The model under review builds one solid part; all positions refer to its coordinate system, in mm. A direction names the side the tool comes from. Give positions to 0.01 mm unless a question says otherwise; leave off trailing zeros. Order: outer loops, then holes, each group sorted by start corner. A loop starts at its lowest first (then second) coordinate and runs counter-clockwise, first axis right, second up. Notation, with made-up numbers: (71, 51) - (78, 51) arc R24 ccw to (78, 64) - close; hole circle Ø5 at (86.25, 75). An arc over 180 degrees is marked (long way). Put each result on its own line as item: value.
```python
from build123d import *

# Parameters (mm, degrees)
SKETCH2_W           = 20
SKETCH2_H           = 77
BOSS_EXTRUDE1_DEPTH = 3
SKETCH3_W           = 15
SKETCH3_H           = 15
BOSS_EXTRUDE2_DEPTH = 3
BOSS_EXTRUDE3_DEPTH = 3
BOSS_EXTRUDE4_DEPTH = 3
SKETCH6_R           = 5
SKETCH6_R_2         = 3
SKETCH6_R_3         = 1.25
CUT_EXTRUDE1_DEPTH  = 4
SKETCH7_R           = 1.25
CUT_EXTRUDE2_DEPTH  = 10


with BuildPart() as part:
    # Sketch2 → Boss-Extrude1 (new body)
    with BuildSketch(Plane.XY):
        with Locations((-46.024750416, 11.319675541)):
            Rectangle(SKETCH2_W, SKETCH2_H)
    extrude(amount=BOSS_EXTRUDE1_DEPTH)

    # Sketch3 → Boss-Extrude2 (add)
    with BuildSketch(Plane.XY.offset(3)):
        with Locations((-63.524750416, 5.819675541)):
            Rectangle(SKETCH3_W, SKETCH3_H)
    extrude(amount=-BOSS_EXTRUDE2_DEPTH)

    # Sketch4 → Boss-Extrude3 (add)
    with BuildSketch(Plane.XY.offset(3)):
        Polygon((-71.024750416, 13.319675541), (-63.524750416, 49.819675541), (-56.024750416, 49.819675541), (-56.024750416, 13.319675541), align=None)
        Polygon((-71.024750416, -1.680324459), (-56.024750416, -27.180324459), (-56.024750416, -1.680324459), align=None)
    extrude(amount=-BOSS_EXTRUDE3_DEPTH)

    # Sketch5 → Boss-Extrude4 (add)
    with BuildSketch(Plane.XY.offset(3)):
        Polygon((-56.024750416, -27.180324459), (-56.024750416, -32.180324459), (-61.024750416, -32.180324459), (-61.024750416, -18.680324459), align=None)
    extrude(amount=-BOSS_EXTRUDE4_DEPTH)

    # Sketch6 → Cut-Extrude1 (cut, through all)
    with BuildSketch(Plane.XY.offset(3)):
        with Locations((-63.524750416, 5.819675541)):
            Circle(SKETCH6_R)
        with Locations((-56.024750416, 30.71445411)):
            Circle(SKETCH6_R_2)
        with Locations((-52.024750416, -22.180324459)):
            Circle(SKETCH6_R_3)
        Polygon((-56.024750416, -27.180324459), (-46.024750416, -23.540622117), (-46.024750416, 49.819675541), (-36.024750416, 49.819675541), (-36.024750416, -27.180324459), (-46.024750416, -27.180324459), align=None)
    extrude(amount=-CUT_EXTRUDE1_DEPTH, mode=Mode.SUBTRACT)

    # Sketch7 → Cut-Extrude2 (cut)
    with BuildSketch(Plane.XY.offset(3)):
        with Locations((-58.774750416, 45.819675541)):
            Circle(SKETCH7_R)
        with Locations((-50.774750416, 45.819675541)):
            Circle(SKETCH7_R)
    extrude(amount=-CUT_EXTRUDE2_DEPTH, mode=Mode.SUBTRACT)


solid = part.part
```
(1) Take a section at A-A, the plane x = -64.5. Write out the cut boundary in (y, z), then the cut area to 3 significant figures.
The answers:
outline: (-12.77, 0) - (0.92, 0) - (0.92, 3) - (-12.77, 3) - close; (10.72, 0) - (45.07, 0) - (45.07, 3) - (10.72, 3) - close
area: 144 mm^2
(2) Take a section at D-D, the plane y = 38. Write out the cut boundary in (x, z).
The answers:
outline: (-65.95, 0) - (-46.02, 0) - (-46.02, 3) - (-65.95, 3) - close
(3) Clearance check with flat-ended pins moving along their axes: pin 1 Ø3.5 at (x, y) = (-56.02, 30.71) entering from -Z; pin 2 Ø1.5 at (x, z) = (-66.5, 1) entering from -Y; pin 3 Ø3 at (x, y) = (-50.77, 45.82) entering from -Z. State where each tip first meets the part, or that it passes through.
The answers:
pin 1: through
pin 2: y = -10.65
pin 3: z = 0
(4) Take a section at C-C, the plane z = 1.05. Write out the cut boundary in (x, y).
The answers:
outline: (-71.02, -1.68) - (-61.02, -18.68) - (-61.02, -32.18) - (-56.02, -32.18) - (-56.02, -27.18) - (-46.02, -23.54) - (-46.02, 49.82) - (-63.52, 49.82) - (-71.02, 13.32) - close; hole circle Ø10 at (-63.52, 5.82); hole circle Ø2.5 at (-58.77, 45.82); hole circle Ø6 at (-56.02, 30.71); hole circle Ø2.5 at (-52.02, -22.18); hole circle Ø2.5 at (-50.77, 45.82)
(5) The part is to be moulded in two halves that separate along X. For faces 1 (the flat face through (-56.025, -30, 2)), 2 (the flat face through (-71.025, 6, 2)), 3 (the cylindrical face through (-58.91, 3.9, 1.52)), 4 (the cylindrical face through (-60.024, 45.875, 1.521)), say which applies: pulls with the +X half, pulls with the -X half, needs draft (parallel to the pull), parting line crosses it, or undercut.
The answers:
face 1: pulls with the +X half
face 2: pulls with the -X half
face 3: undercut
face 4: undercut
(6) Wall thickness on L1, parallel to Y at x = -51.75, z = 0.3; L2, parallel to Y at x = -59.5, z = 1.95; L3, parallel to Y at x = -50.25, z = 1.45: over which ranges is each line inside the solid? List them lowest first.
The answers:
L1: -25.62 to -23.4, -20.96 to 45.04, 46.6 to 49.82
L2: -32.18 to 2.85, 8.79 to 44.8, 46.84 to 49.82
L3: -25.08 to 44.69, 46.95 to 49.82
(7) For faces 5 (the flat face through (-55, 49.82, 2)), 6 (the flat face through (-61.025, -26, 2)), list the 3-axis set-ups (+Z, -Z, +X, -X, +Y, -Y) from which the entire face can be reached by the end or side of a thin tool; tool diameter is ignored.
The answers:
face 5: +Z, -Z, +X, -X, +Y
face 6: +Z, -Z, -X, -Y
(8) Take a section at B-B, the plane y = 29. Write out the cut boundary in (x, z), then the cut area to 3 significant figures.
The answers:
outline: (-67.8, 0) - (-58.49, 0) - (-58.49, 3) - (-67.8, 3) - close; (-53.56, 0) - (-46.02, 0) - (-46.02, 3) - (-53.56, 3) - close
area: 50.6 mm^2
